Input: part model. Units: mm. Frame: model coordinates. A direction names the side the tool comes from. Coordinates: 2 decimals unless noted, no trailing zeros. Order: outer loops, then holes, each group sorted by start corner. A loop starts at its lowest first (then second) coordinate and runs counter-clockwise, first axis right, second up. Notation, with made-up numbers: (-29.75, 38) - (18.25, 38) arc R17 cw to (18.25, 64) - close; hole circle Ø6 at (75.5, -7). An arc over 180 degrees is marked (long way). One line per question, with ' | ' between items.
Autodesk Inventor part; units mm, degrees
ref_plane "YZ Plane" through (0, 0, 0) normal (1, 0, 0) x (0, 1, 0)
ref_plane "XZ Plane" through (0, 0, 0) normal (0, 1, 0) x (-1, 0, 0)
ref_plane "XY Plane" through (0, 0, 0) normal (0, 0, 1) x (1, 0, 0)
sketch "Sketch1" plane through (0, 0, 0) normal (0, 0, 1) x (1, 0, 0)
  line L0 (0, 0) -> (275, 0)
  line L1 (275, 0) -> (275, 10)
  line L2 (0, 0) -> (0, 6)
  line L3 (0, 6) -> (62, 6)
  line L4 (62, 6) -> (66, 10)
  line L5 (275, 10) -> (66, 10)
  dimension "d0" = 275
  dimension "d1" = 10
  dimension "d2" = 6
  dimension "d3" = 62
  dimension "d5" = 135
revolve "Revolution1" add sketch "Sketch1" angle 360 about axis through (0, 0, 0) along (1, 0, 0)
fillet "Fillet1" [suppressed]
fillet "Fillet2" radius 10 1 edges at (275, -10, 0)
fillet "Fillet3" radius 6 1 edges at (0, -6, 0)
properties part number "Tommy Bar"
Item 1: Access query for faces 1 (the face through (164.11, -2.17, 9.76)), 2 (the face through (34, -6, 0)). Directions: +Z, -Z, +X, -X, +Y, -Y. A direction counts if a zero-diameter tool reaches every point of the face in a straight line with its end or side. Return the directions, or none.
Data:
face 1: +X, -X | face 2: -X
Item 2: Section A-A on z = 0. Return the cut outline in (x, y).
Data:
outline: (6, -6) - (62, -6) - (66, -10) - (265, -10) arc R10 ccw to (265, 10) - (66, 10) - (62, 6) - (6, 6) arc R6 ccw to start
Item 3: Contact query for flat-ended pins moving along their axis: P1, Ø3, axis at y = -7, z = -4.5, coming from the +X side; P2, Ø2, axis at x = 114, y = 0.5, coming from the +Z side; P3, Ø3, axis at y = 4, z = -3, coming from the +X side; P4, Ø1.5, axis at x = 89, y = -3, coming from the +Z side. Output: stop coordinate, or through.
Data:
P1: x = 272.31 | P2: z = 10 | P3: x = 274.37 | P4: z = 9.74
Item 4: Section C-C on x = 91.5. Return the cut outline in (y, z), and give its area (3 significant figures).
Data:
outline: circle Ø20 at (0, 0) | area: 314 mm^2
Item 5: Section D-D on x = 27. Return the cut outline in (y, z).
Data:
outline: circle Ø12 at (0, 0)
Item 6: Ray query, line 1 (Z direction, x = 79.5, y = -0.5); line 2 (Z direction, x = 257, y = 1); line 3 (Y direction, x = 202.5, z = 0.75). Return the intervals inside material, ascending.
Data:
line 1: -9.99 to 9.99 | line 2: -9.95 to 9.95 | line 3: -9.97 to 9.97
